Here's how the part is built. I have some questions about the finished solid (model axes, mm). Round coordinates to 2 decimals unless told otherwise and drop trailing zeros. Write each loop counter-clockwise with the first axis right and the second up, starting at its lowest first coordinate (ties: lowest second). Pieces come first, ordered by that corner, then holes. Notation, with made-up numbers: M -30.75,27 L 10.25,27 A3 cw 10.25,31 Z; hole C -39.75,68 d7. An arc over 180 degrees is marked long. Write item = value, one per line. Start each with the question number.
(1) Will this pin go through, and if not, where does the flat tip stop? pin 1 Ø7.5 at (x, z) = (-9.525, 12.7) entering from +Y.
(2) I want a section at C-C (x = -52). List the corners of the cut face in (y, z) for me.
(3) If we mould it in two halves opening along Z, with no side actions, what happens to faces 1 (the cylindrical face through (-0.45, 0.8, 0.48)), 2 (the cylindrical face through (-8.809, 0.783, 15.923)), 3 (the cylindrical face through (-50.676, 0.783, 12.555)), 4 (the flat face through (-31, 0, 13))? For each: released by +Z, released by -Z, zero draft, split by the parting line, or undercut.
(4) I want a section at B-B (y = 0.25). List the corners of the cut face in (x, z) for me (1 decimal).
(5) I need wall thicknesses on line 1 along X through (y, z) = (1.35, 13); line 2 along X through (y, z) = (0.4, 11.5); line 3 along Z through (x, y) = (-6.5, 0.75). Which ranges of each line are inside material? Lowest first, please.
(6) I want a section at A-A (z = 12.7). List the corners of the cut face in (x, y) for me, and give its area (3 significant figures).
Autodesk Inventor part; units mm, degrees
ref_plane "YZ Plane" through (0, 0, 0) normal (1, 0, 0) x (0, 1, 0)
ref_plane "XZ Plane" through (0, 0, 0) normal (0, 1, 0) x (-1, 0, 0)
ref_plane "XY Plane" through (0, 0, 0) normal (0, 0, 1) x (1, 0, 0)
sketch "Sketch1" plane through (0, 0, 0) normal (0, 1, 0) x (-1, 0, 0)
  line L0 (0, 0) -> (63.5, 0)
  line L1 (63.5, 0) -> (63.5, 25.4)
  line L2 (63.5, 25.4) -> (0, 25.4)
  line L3 (0, 25.4) -> (0, 0)
  circle A0 centre (9.525, 12.7) radius 3.302
  circle A1 centre (53.975, 12.7) radius 3.302
  line L4 (9.525, 12.7) -> (53.975, 12.7) construction
  line L5 (31.75, 25.4) -> (31.75, 0) construction
  point P0 (31.75, 12.7)
  dimension "d0" = 63.5
  dimension "d2" = 25.4
  dimension "d3" = 44.45
  dimension "d4" = 6.604
extrude "Extrusion1" add sketch "Sketch1" along normal blind 1.5875
fillet "Fillet1" radius 1.5875 4 edges at (0, 0.7937, 25.4) (0, 0.7937, 0) (-63.5, 0.7937, 0) (-63.5, 0.7937, 25.4)
properties part number "Wheel Drop Down Plate" material "Aluminum 6061"
Returned:
q1.pin_1 = 1.59
q2.outline = M 0,0 L 1.59,0 L 1.59,10.05 L 0,10.05 Z; M 0,15.35 L 1.59,15.35 L 1.59,25.4 L 0,25.4 Z
q3.face_1 = released by -Z
q3.face_2 = undercut
q3.face_3 = undercut
q3.face_4 = zero draft
q4.outline = M -63.5,1.6 A1.6 ccw -61.9,0 L -1.6,0 A1.6 ccw 0,1.6 L 0,23.8 A1.6 ccw -1.6,25.4 L -61.9,25.4 A1.6 ccw -63.5,23.8 Z; hole C -54,12.7 d6.6; hole C -9.5,12.7 d6.6
q5.line_1 = -63.5 to -57.26, -50.69 to -12.81, -6.24 to 0
q5.line_2 = -63.5 to -57.05, -50.9 to -12.6, -6.45 to 0
q5.line_3 = 0 to 11.38, 14.02 to 25.4
q6.outline = M -63.5,0 L -57.28,0 L -57.28,1.59 L -63.5,1.59 Z; M -50.67,0 L -12.83,0 L -12.83,1.59 L -50.67,1.59 Z; M -6.22,0 L 0,0 L 0,1.59 L -6.22,1.59 Z
q6.area = 79.8 mm²
